from build123d import *

# Parameters (mm, degrees)
SKETCH_1_R          = 9.7
EXTRUDE_1_DEPTH     = 4
SKETCH_2_R          = 1
CUT_EXTRUDE_1_DEPTH = 10
CUT_EXTRUDE_2_DEPTH = 10
SKETCH_4_R          = 1
CUT_EXTRUDE_3_DEPTH = 10


with BuildPart() as part:
    # 草图1 → 凸台-拉伸1 (new body)
    with BuildSketch(Plane.XY):
        with BuildLine():
            Line((0, 19.7), (250, 19.7))
            ThreePointArc((250, 19.7), (269.7, 0), (250, -19.7))
            Line((250, -19.7), (0, -19.7))
            ThreePointArc((0, -19.7), (-19.7, 0), (0, 19.7))
        make_face()
        Circle(SKETCH_1_R, mode=Mode.SUBTRACT)
        with Locations((250, 0)):
            Circle(SKETCH_1_R, mode=Mode.SUBTRACT)
    extrude(amount=EXTRUDE_1_DEPTH)

    # 草图2 → 切除-拉伸1 (cut)
    with BuildSketch(Plane.XY.offset(4)):
        with Locations((25, 15)):
            Circle(SKETCH_2_R)
        with Locations((90, 15)):
            Circle(SKETCH_2_R)
        with Locations((155, 15)):
            Circle(SKETCH_2_R)
        with Locations((220, 15)):
            Circle(SKETCH_2_R)
        with Locations((90, -15)):
            Circle(SKETCH_2_R)
        with Locations((155, -15)):
            Circle(SKETCH_2_R)
        with Locations((220, -15)):
            Circle(SKETCH_2_R)
        with Locations((25, -15)):
            Circle(SKETCH_2_R)
    extrude(amount=-CUT_EXTRUDE_1_DEPTH, mode=Mode.SUBTRACT)

    # 草图3 → 切除-拉伸2 (cut)
    with BuildSketch(Plane.XY.offset(4)):
        with BuildLine():
            Line((32, 8), (114.023268405, 8))
            ThreePointArc((114.023268405, 8), (115.976706085, 6.429046887), (114.86138476, 4.184081231))
            Line((114.86138476, 4.184081231), (88.462542093, -8))
            Line((88.462542093, -8), (32, -8))
            Line((32, -8), (32, 8))
        make_face()
        with BuildLine():
            Line((156.537457907, 8), (130.13861524, -4.184081231))
            ThreePointArc((130.13861524, -4.184081231), (129.023293915, -6.429046887), (130.976731595, -8))
            Line((130.976731595, -8), (213, -8))
            Line((213, -8), (213, 8))
            Line((213, 8), (156.537457907, 8))
        make_face()
    extrude(amount=-CUT_EXTRUDE_2_DEPTH, mode=Mode.SUBTRACT)

    # 草图4 → 切除-拉伸3 (cut)
    with BuildSketch(Plane.XY.offset(4)):
        with Locations((0, 9.7)):
            Circle(SKETCH_4_R)
        with Locations((250, 9.7)):
            Circle(SKETCH_4_R)
    extrude(amount=-CUT_EXTRUDE_3_DEPTH, mode=Mode.SUBTRACT)


solid = part.part
Can you work these out from the model? Positions are in its coordinate system, mm. A direction names the side the tool comes from. Give positions to 0.01 mm unless a question says otherwise; leave off trailing zeros. Order: outer loops, then holes, each group sorted by start corner. A loop starts at its lowest first (then second) coordinate and runs counter-clockwise, first axis right, second up. Notation, with made-up numbers: M 41.5,62.25 L 76.5,62.25 A28 cw 76.5,89.25 Z; hole C 81.25,-22 d4. An arc over 180 degrees is marked long. Use one line per item in the form item = value. Start each with the question number.
Item 1: Will these pins go through, and if not, where does the flat tip stop? pin 1 Ø1.2 at (y, z) = (-1.5, 2.5) entering from +X; pin 2 Ø2 at (y, z) = (-2.5, 1.5) entering from -X.
Item 2: If we section it at A-A (x = 192): Write out the boundary of the cut face in (y, z), then the cut area to 3 significant figures.
Item 3: If we section it at C-C (y = 0): Write out the boundary of the cut face in (x, z).
Item 4: We'd pull the mould along X, two halves only. Please class faces 3 (the cylindrical face through (249.59, -9.69, 1.97)), 4 (the cylindrical face through (-19.695, -0.433, 1.972)), 5 (the flat face through (127, 0, 0)): +X half, -X half, draft (parallel to the pull), parting line (faces both ways), or undercut.
Item 5: If we section it at D-D (x = 100): Write out the boundary of the cut face in (y, z).
Item 6: If we section it at B-B (z = 1.05): State how many separate pieces and enclosed holes the cut face has, then the cut area to 3 significant figures.
Item 7: For faces 1 (the flat face through (143.52, 1.99, 2.03)), 2 (the cylindrical face through (269.695, 0.433, 1.972)), which set-ups out of +Z, -Z, +X, -X, +Y, -Y let a thin tool reach every point of the face, with its end or its side?
Item 8: If I drill on line 1 along Y through (x, z) = (220, 1.3); line 2 along Y through (x, z) = (45.5, 3.8); line 3 along Y through (x, z) = (155, 1.3), over which ranges is the centre line in solid material (lowest first)?
Outcome:
q1.pin_1 = 269.68
q1.pin_2 = -19.64
q2.outline = M -19.7,0 L -8,0 L -8,4 L -19.7,4 Z; M 8,0 L 19.7,0 L 19.7,4 L 8,4 Z
q2.area = 93.6 mm2
q3.outline = M -19.7,0 L -9.7,0 L -9.7,4 L -19.7,4 Z; M 9.7,0 L 32,0 L 32,4 L 9.7,4 Z; M 105.8,0 L 139.2,0 L 139.2,4 L 105.8,4 Z; M 213,0 L 240.3,0 L 240.3,4 L 213,4 Z; M 259.7,0 L 269.7,0 L 269.7,4 L 259.7,4 Z
q4.face_3 = undercut
q4.face_4 = -X half
q4.face_5 = draft
q5.outline = M -19.7,0 L -2.68,0 L -2.68,4 L -19.7,4 Z; M 8,0 L 19.7,0 L 19.7,4 L 8,4 Z
q6.separate_pieces = 1
q6.enclosed_holes = 12
q6.area = 8,110 mm2
q7.face_1 = +Z, -Z
q7.face_2 = +Z, -Z, +X
q8.line_1 = -19.7 to -16, -14 to 14, 16 to 19.7
q8.line_2 = -19.7 to -8, 8 to 19.7
q8.line_3 = -19.7 to -16, -14 to -8, 7.29 to 14, 16 to 19.7
